from build123d import *

# Parameters (mm, degrees)
SKETCH1_W           = 38.1
SKETCH1_H           = 37.084
BOSS_EXTRUDE1_DEPTH = 4.826
SKETCH3_R           = 1.27
CUT_EXTRUDE2_DEPTH  = 54.386546358
CUT_EXTRUDE3_DEPTH  = 54.386546358
SKETCH5_W           = 7.62
SKETCH5_H           = 3.409901171
CUT_EXTRUDE4_DEPTH  = 54.386546358
SKETCH7_W           = 4.826
SKETCH7_H           = 6.380433542
SKETCH7_H_2         = 6.35
CUT_EXTRUDE5_DEPTH  = 54.386546358


with BuildPart() as part:
    # Sketch1 → Boss-Extrude1 (new body)
    with BuildSketch(Plane.XY):
        with Locations((19.05, 18.542)):
            Rectangle(SKETCH1_W, SKETCH1_H)
    extrude(amount=BOSS_EXTRUDE1_DEPTH)

    # Sketch3 → Cut-Extrude2 (cut, through all)
    with BuildSketch(Plane.XY.offset(4.826)):
        with Locations((2.580480538, 6.0325)):
            Circle(SKETCH3_R)
        with Locations((31.836519462, 6.0325)):
            Circle(SKETCH3_R)
    extrude(amount=-CUT_EXTRUDE2_DEPTH, mode=Mode.SUBTRACT)

    # Sketch4 → Cut-Extrude3 (cut, through all)
    with BuildSketch(Plane(origin=(0, 0, 0), x_dir=(-1, 0, 0), z_dir=(0, 0, -1))):
        with BuildLine():
            Line((-28.702, 12.065), (-5.715, 12.065))
            ThreePointArc((-5.715, 12.065), (-5.625197439, 12.027802561), (-5.588, 11.938))
            Line((-5.588, 11.938), (-5.588, 0.127))
            ThreePointArc((-5.588, 0.127), (-5.625197439, 0.037197439), (-5.715, 0))
            Line((-5.715, 0), (-28.702, 0))
            ThreePointArc((-28.702, 0), (-28.791802561, 0.037197439), (-28.829, 0.127))
            Line((-28.829, 0.127), (-28.829, 11.938))
            ThreePointArc((-28.829, 11.938), (-28.791802561, 12.027802561), (-28.702, 12.065))
        make_face()
    extrude(amount=-CUT_EXTRUDE3_DEPTH, mode=Mode.SUBTRACT)

    # Sketch5 → Cut-Extrude4 (cut, through all)
    with BuildSketch(Plane.XY.offset(4.826)):
        with Locations((11.43, 35.379049415)):
            Rectangle(SKETCH5_W, SKETCH5_H)
        with Locations((26.67, 35.379049415)):
            Rectangle(SKETCH5_W, SKETCH5_H)
    extrude(amount=-CUT_EXTRUDE4_DEPTH, mode=Mode.SUBTRACT)

    # Sketch7 → Cut-Extrude5 (cut, through all)
    with BuildSketch(Plane.XY.offset(4.826)):
        with Locations((2.413, 24.1643156)):
            Rectangle(SKETCH7_W, SKETCH7_H)
        with Locations((35.687, 24.149098829)):
            Rectangle(SKETCH7_W, SKETCH7_H_2)
    extrude(amount=-CUT_EXTRUDE5_DEPTH, mode=Mode.SUBTRACT)


solid = part.part
Verification items for the finished model (mm, model axes). A direction names the side the tool comes from. Round coordinates to 2 decimals unless told otherwise and drop trailing zeros. Loops run counter-clockwise (first coordinate to the right, second up) from the corner with the lowest first, then second, coordinate; pieces in that order, holes last. Notation, with made-up numbers: (-16.75, -30.5) - (22.25, -30.5) arc R33 cw to (22.25, 2.5) - close; hole circle Ø3 at (-39.75, 35). An arc over 180 degrees is marked (long way). Use a Markdown table: item, result. Add a question column.
1. Section check D-D, the plane z = 1.85. Give the number of separate pieces and of enclosed holes in the cut face, plus the area to 3 significant figures.
2. Section check B-B, the plane x = 34.5. Record the boundary of the cut face in (y, z).
3. Section check C-C, the plane y = 35.5. Record the boundary of the cut face in (x, z).
4. Gauge pin test, flat ends, axial feed: pin 1 (2 mm diameter, centred on x = 8, z = 1.5, fed in from -Y) (3 decimals); pin 2 (1.4 mm diameter, centred on x = 13, z = 1.5, fed in from +Y); pin 3 (1.4 mm diameter, centred on y = 24, z = 3, fed in from -X). Record the tip position at first contact, or that the pin passes through.
5. Section check A-A, the plane y = 11. Record the boundary of the cut face in (x, z).
6. Release check for a two-part mould opening along Y. For faces 6 (the face through (38.1, 10, 2)), 7 (the face through (2, 27.355, 2)), 8 (the face through (33, 0, 2)) record: released by +Y, released by -Y, zero draft, split by the parting line, or undercut.
7. Access from +Z, -Z, +X, -X, +Y, -Y to the whole of each face (thin tool, end or side, straight path). Record for faces 1 (the face through (19, 23, 4.826)), 2 (the face through (36, 20.974, 2)), 3 (the face through (30.48, 35, 2)), 4 (the face through (28.829, 6, 2)), 5 (the face through (4.826, 24, 2)).
8. Thickness scan on probe 1 along X at (y, z) = (35, 0.4); probe 2 along X at (y, z) = (3, 3.7); probe 3 along Y at (x, z) = (13.5, 3.65) (3 decimals). Record the ranges inside material, lowest first. Write a range as [from, to].
Checks:
| question | item | result |
|---|---|---|
| 1 | separate pieces | 1 |
| 1 | enclosed holes | 2 |
| 1 | area | 1,010 mm^2 |
| 2 | outline | (0, 0) - (20.97, 0) - (20.97, 4.83) - (0, 4.83) - close; (27.32, 0) - (37.08, 0) - (37.08, 4.83) - (27.32, 4.83) - close |
| 3 | outline | (0, 0) - (7.62, 0) - (7.62, 4.83) - (0, 4.83) - close; (15.24, 0) - (22.86, 0) - (22.86, 4.83) - (15.24, 4.83) - close; (30.48, 0) - (38.1, 0) - (38.1, 4.83) - (30.48, 4.83) - close |
| 4 | pin 1 | stops at y = 12.065 |
| 4 | pin 2 | stops at y = 33.67 |
| 4 | pin 3 | stops at x = 4.83 |
| 5 | outline | (0, 0) - (5.59, 0) - (5.59, 4.83) - (0, 4.83) - close; (28.83, 0) - (38.1, 0) - (38.1, 4.83) - (28.83, 4.83) - close |
| 6 | face 6 | zero draft |
| 6 | face 7 | undercut |
| 6 | face 8 | released by -Y |
| 7 | face 1 | +Z, +X, -X, +Y, -Y |
| 7 | face 2 | +Z, -Z, +X |
| 7 | face 3 | +Z, -Z, +Y |
| 7 | face 4 | +Z, -Z |
| 7 | face 5 | +Z, -Z, -X |
| 8 | probe 1 | x = [0, 7.62], [15.24, 22.86], [30.48, 38.1] |
| 8 | probe 2 | x = [0, 5.59], [28.83, 38.1] |
| 8 | probe 3 | y = [12.065, 33.674] |
